```python
from build123d import *

# Parameters (mm, degrees)
F1_DEPTH = 20


with BuildPart() as f1:
    # F0 (on Top) → F1 (new body)
    with BuildSketch(Plane.XY):
        with BuildLine():
            ThreePointArc((40, 187), (10.111843, 95.615114), (0, 0))
            Line((0, 0), (100, 0))
            Line((100, 0), (100, 145))
            Line((100, 145), (40, 187))
        make_face()
        with BuildLine():
            Line((100, 0), (0, 0))
            ThreePointArc((0, 0), (10.111843, -95.615114), (40, -187))
            Line((40, -187), (100, -145))
            Line((100, -145), (100, 0))
        make_face()
        with BuildLine():
            Line((100, 145), (100, 0))
            Line((100, 0), (183, 0))
            Line((183, 0), (183, 125))
            add(Edge.make_bspline(
                [(100, 145), (123.31415, 128.680095), (155.358294, 118.230603), (183, 125)],
                knots=[0, 0, 0, 0, 85.375641, 85.375641, 85.375641, 85.375641], degree=3))
        make_face()
        with BuildLine():
            Line((183, 0), (100, 0))
            Line((100, 0), (100, -145))
            add(Edge.make_bspline(
                [(100, -145), (123.31415, -128.680095), (155.358294, -118.230603), (183, -125)],
                knots=[0, 0, 0, 0, 85.375641, 85.375641, 85.375641, 85.375641], degree=3))
            Line((183, -125), (183, 0))
        make_face()
        Polygon((183, 125), (183, 0), (330, 0), (330, 161), align=None)
        Polygon((330, 0), (183, 0), (183, -125), (330, -161), align=None)
        with BuildLine():
            Line((330, 161), (330, 0))
            Line((330, 0), (474, 0))
            Line((474, 0), (474, 158))
            ThreePointArc((474, 158), (402.196918, 168.952057), (330, 161))
        make_face()
        with BuildLine():
            Line((474, 0), (330, 0))
            Line((330, 0), (330, -161))
            ThreePointArc((330, -161), (402.196918, -168.952057), (474, -158))
            Line((474, -158), (474, 0))
        make_face()
        with BuildLine():
            Line((474, 158), (474, 0))
            Line((474, 0), (587.999996, 0))
            Line((587.999996, 0), (587.999996, 203))
            add(Edge.make_bspline(
                [(474, 158), (498.337581, 150.951675), (536.193063, 151.193067), (587.999996, 203)],
                knots=[0, 0, 0, 0, 122.560186, 122.560186, 122.560186, 122.560186], degree=3))
        make_face()
        with BuildLine():
            Line((587.999996, 0), (474, 0))
            Line((474, 0), (474, -158))
            add(Edge.make_bspline(
                [(474, -158), (498.337581, -150.951675), (536.193063, -151.193067), (587.999996, -203)],
                knots=[0, 0, 0, 0, 122.560186, 122.560186, 122.560186, 122.560186], degree=3))
            Line((587.999996, -203), (587.999996, 0))
        make_face()
        with BuildLine():
            Line((587.999996, 203), (587.999996, 0))
            Line((587.999996, 0), (642.999996, 0))
            Line((642.999996, 0), (642.999996, 207))
            ThreePointArc((642.999996, 207), (615.543759, 204.398263), (587.999996, 203))
        make_face()
        with BuildLine():
            Line((642.999996, 0), (587.999996, 0))
            Line((587.999996, 0), (587.999996, -203))
            ThreePointArc((587.999996, -203), (615.543759, -204.398263), (642.999996, -207))
            Line((642.999996, -207), (642.999996, 0))
        make_face()
        Polygon((642.999996, 207), (642.999996, 0), (720.000004, 0), (720.000004, 216), align=None)
        Polygon((720.000004, 0), (642.999996, 0), (642.999996, -207), (720.000004, -216), align=None)
        with BuildLine():
            Line((720.000004, 216), (720.000004, 0))
            Line((720.000004, 0), (820, 0))
            Line((820, 0), (820, 207))
            ThreePointArc((820, 207), (770.465406, 216.671153), (720.000004, 216))
        make_face()
        with BuildLine():
            Line((820, 0), (720.000004, 0))
            Line((720.000004, 0), (720.000004, -216))
            ThreePointArc((720.000004, -216), (770.465406, -216.671153), (820, -207))
            Line((820, -207), (820, 0))
        make_face()
    extrude(amount=F1_DEPTH)


solid = f1.part
```
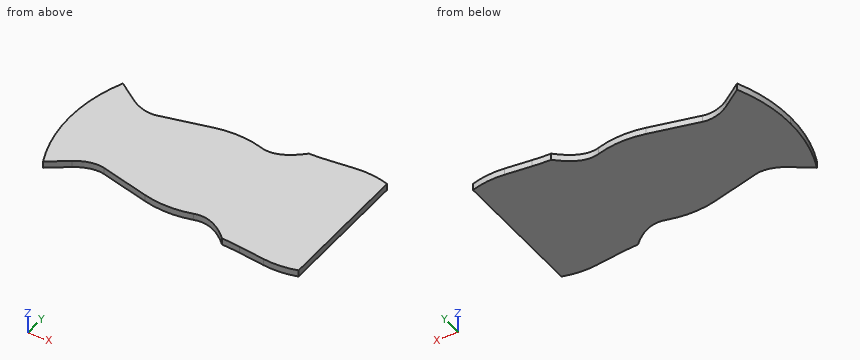
Build history of the part. All positions in model axes, mm. Give positions to 0.01 mm unless a question says otherwise; leave off trailing zeros. Order: outer loops, then holes, each group sorted by start corner. A loop starts at its lowest first (then second) coordinate and runs counter-clockwise, first axis right, second up. Notation, with made-up numbers: M 4.25,56 L 56.25,56 A29 cw 56.25,87 Z; hole C -25.5,22.5 d8. An arc over 180 degrees is marked long. Write item = value, one per line. Start each with the question number.
(1) Probe L1, parallel to X at y = 184.5, z = 2; L2, parallel to X at y = 179, z = 5.75; L3, parallel to X at y = 2, z = 5.5. List the from-to ranges inside material, lowest first. Write a range as [from, to].
(2) Pin check, flat tips, straight feed: pin 1 Ø12 at (x, z) = (104, 10.5) entering from +Y; pin 2 Ø10 at (x, z) = (322.5, 10) entering from -Y; pin 3 Ø1 at (y, z) = (-102.5, 17) entering from -X. Stop position of each tip, or through.
(3) Slice it at B-B on x = 304.5. Write the cut outline in (y, z).
(4) Slice it at A-A on x = 71. Write the cut outline in (y, z).
Responses:
q1.L1 = [38.89, 43.57], [567.5, 820]
q1.L2 = [36.5, 51.43], [560.32, 820]
q1.L3 = [0, 820]
q2.pin_1 = 146.4
q2.pin_2 = -160.39
q2.pin_3 = 11.53
q3.outline = M -154.76,0 L 154.76,0 L 154.76,20 L -154.76,20 Z
q4.outline = M -165.3,0 L 165.3,0 L 165.3,20 L -165.3,20 Z
